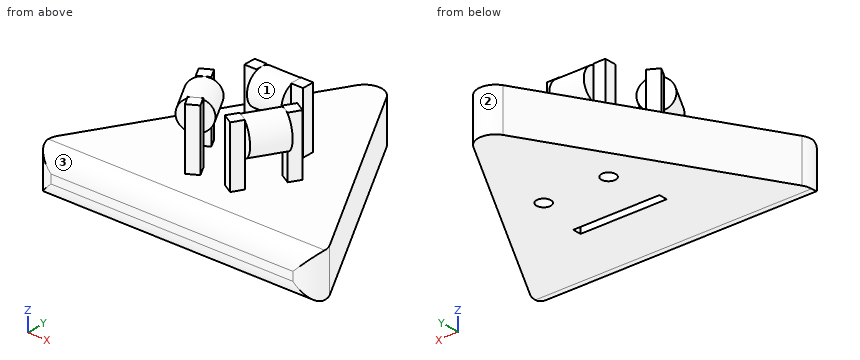
from build123d import *

# Parameters (mm, degrees)
EXTRUDE_1_DEPTH        = 10
FILLET_1_R             = 4
SKETCH_2_W             = 2.8
SKETCH_2_H             = 2.8
EXTRUDE_2_DEPTH        = 14
SKETCH_3_R             = 3.6
EXTRUDE_3_DEPTH        = 8
SKETCH_4_R             = 4
EXTRUDE_4_DEPTH        = 8
SKETCH_5_R             = 4
EXTRUDE_5_DEPTH        = 8
SKETCH_6_W             = 20
SKETCH_6_H             = 2
CUT_EXTRUDE_1_DEPTH    = 8
HOLE_WIZARD_M4_1_D     = 3.3
HOLE_WIZARD_M4_1_DEPTH = 5
HOLE_WIZARD_M4_1_TIP   = 0.991420021


with BuildPart() as part:
    # 草图1 → 凸台-拉伸1 (new body)
    with BuildSketch(Plane.XY):
        Polygon((0, 40), (35, -20.621778265), (-35, -20.621778265), align=None)
    extrude(amount=EXTRUDE_1_DEPTH)

    # 圆角1
    fillet_1_edges = [part.edges().sort_by_distance(p)[0] for p in [
        (0, -20.621778265, 10),
        (0, -20.621778265, 0),
        (35, -20.621778265, 5),
        (-35, -20.621778265, 5),
        (0, 40, 5),
    ]]
    fillet(fillet_1_edges, radius=FILLET_1_R)

    # 草图2 → 凸台-拉伸2 (add)
    with BuildSketch(Plane.XY.offset(10)):
        with Locations((-5.4, 8.6)):
            Rectangle(SKETCH_2_W, SKETCH_2_H)
        with Locations((5.4, 8.6)):
            Rectangle(SKETCH_2_W, SKETCH_2_H)
        Polygon((10.660254038, -1.535898385), (12.060254038, 0.888972746), (9.635382907, 2.288972746), (8.235382907, -0.135898385), align=None)
        Polygon((5.260254038, -10.888972746), (2.835382907, -9.488972746), (4.235382907, -7.064101615), (6.660254038, -8.464101615), align=None)
        Polygon((-6.660254038, -8.464101615), (-5.260254038, -10.888972746), (-2.835382907, -9.488972746), (-4.235382907, -7.064101615), align=None)
        Polygon((-12.060254038, 0.888972746), (-9.635382907, 2.288972746), (-8.235382907, -0.135898385), (-10.660254038, -1.535898385), align=None)
    extrude(amount=EXTRUDE_2_DEPTH)

    # 草图3 → 凸台-拉伸3 (add)
    with BuildSketch(Plane(origin=(-2, 3.464101615, 0), x_dir=(-0.866025404, -0.5, 0), z_dir=(0.5, -0.866025404, 0))):
        with Locations((8.6, -20.4)):
            Circle(SKETCH_3_R)
    extrude(amount=EXTRUDE_3_DEPTH)

    # 草图4 → 凸台-拉伸4 (add)
    with BuildSketch(Plane(origin=(-4, 0, 0), x_dir=(0, 0, -1), z_dir=(1, 0, 0))):
        with Locations((-20, 8.6)):
            Circle(SKETCH_4_R)
    extrude(amount=EXTRUDE_4_DEPTH)

    # 草图5 → 凸台-拉伸5 (add)
    with BuildSketch(Plane(origin=(2, 3.464101615, 0), x_dir=(-0.866025404, 0.5, 0), z_dir=(-0.5, -0.866025404, 0))):
        with Locations((-8.6, -20)):
            Circle(SKETCH_5_R)
    extrude(amount=EXTRUDE_5_DEPTH)

    # 草图6 → 切除-拉伸1 (cut)
    with BuildSketch(Plane(origin=(0, 0, 0), x_dir=(-1, 0, 0), z_dir=(0, 0, -1))):
        with Locations((0, -2)):
            Rectangle(SKETCH_6_W, SKETCH_6_H)
    extrude(amount=-CUT_EXTRUDE_1_DEPTH, mode=Mode.SUBTRACT)

    # M4 螺纹孔1
    with Locations(Plane(origin=(0, 0, 0), x_dir=(-1, 0, 0), z_dir=(0, 0, -1))):
        with Locations((-7.497367874, 10.020225249), (7.560370965, 10.020225249)):
            Hole(HOLE_WIZARD_M4_1_D / 2, depth=HOLE_WIZARD_M4_1_DEPTH)
            with Locations((0, 0, -(HOLE_WIZARD_M4_1_DEPTH + HOLE_WIZARD_M4_1_TIP / 2))):  # 118° drill point
                Cone(0, HOLE_WIZARD_M4_1_D / 2, HOLE_WIZARD_M4_1_TIP, mode=Mode.SUBTRACT)


solid = part.part
Could you check a few things on this model? Use its own coordinates, in mm. Face numbers are marked on the shaded views. Give positions to 0.01 mm unless a question says otherwise; leave off trailing zeros. Order: outer loops, then holes, each group sorted by start corner. A loop starts at its lowest first (then second) coordinate and runs counter-clockwise, first axis right, second up. Notation, with made-up numbers: (-3, 61) - (42, 61) arc R26 cw to (42, 87) - close; hole circle Ø2 at (-9, -16). An arc over 180 degrees is marked (long way). One line per item, written item: value. Start each with the question number.
1. Imagine slicing it at C-C on y = 19.5. List the corners of the cut face in (x, z) for me.
2. Imagine slicing it at B-B on x = 23. List the corners of the cut face in (y, z) for me.
3. Thinking about a two-plate mould opening in Z: for the marked faces 1, 2 and 3, which applies, +Z half, -Z half, draft (parallel to the pull), parting line (faces both ways), or undercut?
4. Imagine slicing it at D-D on y = 32.5. List the corners of the cut face in (x, z) for me.
5. Imagine slicing it at A-A on z = 11.75. List the corners of the cut face in (x, y) for me, plus the area to 3 significant figures.
6. If I drill on probe 1 along Z at (x, y) = (15.5, 5); probe 2 along Z at (x, y) = (-4.5, -7); probe 3 along Y at (x, z) = (-11, 18.5), over which ranges is the centre line in solid material (lowest first)?
7. For P1, Ø10, axis at x = 8, z = 11.5, coming from the -Y side; P2, Ø10, axis at x = -22, z = 17.5, coming from the +Y side; P3, Ø2, axis at x = -6, z = 15, coming from the -Y side; P4, Ø4, axis at x = -13.5, z = 10.5, coming from the +Y side, each with a flat end and sliding along its axis, tell me the tip position at first contact or that it passes through.
Values:
1. outline: (-11.84, 0) - (11.84, 0) - (11.84, 10) - (-11.84, 10) - close
2. outline: (-20.62, 4) arc R4 ccw to (-16.62, 0) - (0.16, 0) - (0.16, 10) - (-16.62, 10) arc R4 ccw to (-20.62, 6) - close
3. face 1: undercut
3. face 2: draft
3. face 3: +Z half
4. outline: (-4.33, 0) - (4.33, 0) - (4.33, 10) - (-4.33, 10) - close
5. outline: (-12.06, 0.89) - (-10.66, -1.54) - (-8.24, -0.14) - (-9.64, 2.29) - close; (-6.8, 7.2) - (-4, 7.2) - (-4, 10) - (-6.8, 10) - close; (-6.66, -8.46) - (-5.26, -10.89) - (-2.84, -9.49) - (-4.24, -7.06) - close; (2.84, -9.49) - (5.26, -10.89) - (6.66, -8.46) - (4.24, -7.06) - close; (4, 7.2) - (6.8, 7.2) - (6.8, 10) - (4, 10) - close; (8.24, -0.14) - (10.66, -1.54) - (12.06, 0.89) - (9.64, 2.29) - close
5. area: 47.0 mm²
6. probe 1: 0 to 10
6. probe 2: 0 to 10, 17.01 to 23.79
6. probe 3: -4.26 to -1.73, -0.95 to 1.5
7. P1: y = -20.59
7. P2: through
7. P3: y = -10.89
7. P4: y = 19.97
